from build123d import *

# Parameters (mm, degrees)
SKETCH2_R           = 1.55
BOSS_EXTRUDE1_DEPTH = 7.5
SKETCH4_W           = 8
SKETCH4_H           = 1.5
BOSS_EXTRUDE3_DEPTH = 20
SKETCH5_R           = 1.55
BOSS_EXTRUDE4_DEPTH = 7.5
SKETCH6_W           = 0.75
SKETCH6_H           = 0.5
CUT_EXTRUDE1_DEPTH  = 9
SKETCH7_R           = 1.1
CUT_EXTRUDE2_DEPTH  = 3.5
CHAMFER1_SIZE       = 1.1
FILLET1_R           = 3


with BuildPart() as part:
    # Sketch2 → Boss-Extrude1 (new body)
    with BuildSketch(Plane.XY):
        with BuildLine():
            Line((3.05, 2.05), (11.05, 2.05))
            Line((11.05, 2.05), (11.05, 0.55))
            Line((11.05, 0.55), (3.05, 0.55))
            Line((3.05, 0.55), (3.05, 0))
            ThreePointArc((3.05, 0), (0, -3.05), (-3.05, 0))
            Line((-3.05, 0), (-3.05, 2.05))
            Line((-3.05, 2.05), (-2.258317958, 2.05))
            ThreePointArc((-2.258317958, 2.05), (-1.234908904, 2.788816953), (0, 3.05))
            Line((0, 3.05), (3.05, 3.05))
            Line((3.05, 3.05), (3.05, 2.05))
        make_face()
        Circle(SKETCH2_R, mode=Mode.SUBTRACT)
    extrude(amount=BOSS_EXTRUDE1_DEPTH)

    # Sketch4 → Boss-Extrude3 (add)
    with BuildSketch(Plane.XY.offset(7.5)):
        with Locations((7.05, 1.3)):
            Rectangle(SKETCH4_W, SKETCH4_H)
    extrude(amount=BOSS_EXTRUDE3_DEPTH)

    # Sketch5 → Boss-Extrude4 (add)
    with BuildSketch(Plane.XY.offset(27.5)):
        with BuildLine():
            Line((11.05, 0.55), (11.05, 2.05))
            Line((11.05, 2.05), (3.05, 2.05))
            Line((3.05, 2.05), (3.05, 3.05))
            Line((3.05, 3.05), (0, 3.05))
            ThreePointArc((0, 3.05), (-1.234908904, 2.788816953), (-2.258317958, 2.05))
            Line((-2.258317958, 2.05), (-3.05, 2.05))
            Line((-3.05, 2.05), (-3.05, 0))
            ThreePointArc((-3.05, 0), (0, -3.05), (3.05, 0))
            Line((3.05, 0), (3.05, 0.55))
            Line((3.05, 0.55), (11.05, 0.55))
        make_face()
        Circle(SKETCH5_R, mode=Mode.SUBTRACT)
    extrude(amount=BOSS_EXTRUDE4_DEPTH)

    # Sketch6 → Cut-Extrude1 (cut, through all)
    with BuildSketch(Plane.ZY.offset(-3.05)):
        with Locations((19.4, 1.8)):
            Rectangle(SKETCH6_W, SKETCH6_H)
    extrude(amount=-CUT_EXTRUDE1_DEPTH, mode=Mode.SUBTRACT)

    # Sketch7 → Cut-Extrude2 (cut, through all)
    with BuildSketch(Plane.XZ.offset(-0.55)):
        with Locations((7.05, 25)):
            Circle(SKETCH7_R)
        with Locations((7.05, 10)):
            Circle(SKETCH7_R)
        with Locations((7.05, 31)):
            Circle(SKETCH7_R)
        with Locations((7.05, 4)):
            Circle(SKETCH7_R)
    extrude(amount=-CUT_EXTRUDE2_DEPTH, mode=Mode.SUBTRACT)

    # Chamfer1
    chamfer1_edges = [part.edges().sort_by_distance(p)[0] for p in [
        (5.95, 0.55, 10),
        (5.95, 0.55, 25),
        (5.95, 0.55, 4),
        (5.95, 0.55, 31),
    ]]
    chamfer(chamfer1_edges, length=CHAMFER1_SIZE)

    # Fillet1
    fillet1_edges = [part.edges().sort_by_distance(p)[0] for p in [
        (11.05, 1.3, 0),
        (11.05, 1.3, 35),
    ]]
    fillet(fillet1_edges, radius=FILLET1_R)


solid = part.part
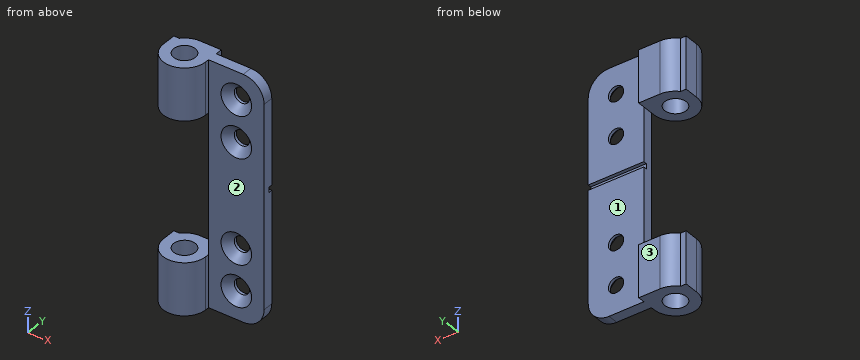
Source: CAD feature listing. Evaluate the final solid. Frame: model axes, mm. Face numbers are marked on the shaded views. A direction names the side the tool comes from. Give positions to 0.01 mm unless a question says otherwise; leave off trailing zeros. Loops run counter-clockwise (first coordinate to the right, second up) from the corner with the lowest first, then second, coordinate; pieces in that order, holes last. Notation, with made-up numbers: (-14, -38) -> (25, -38) arc R26 cw to (25, -14) -> close; hole circle Ø2 at (-25, 65.5). An arc over 180 degrees is marked (long way). Use a Markdown table: item, result. Add a question column.
1) First-contact query: pin 1 (0.8 mm diameter, centred on y = 3, z = 32, fed in from +X); pin 2 (6.5 mm diameter, centred on x = 8, z = 11.5, fed in from +Y); pin 3 (4 mm diameter, centred on x = 7.5, z = 11.5, fed in from -Y); pin 4 (1.9 mm diameter, centred on x = 0, y = 0, fed in from +Z). Flat tips, straight axial feed; report the tip coordinate or a pass-through.
2) Section query B-B, the plane x = 7.05. Count the separate pieces of the cut face and the enclosed holes in it, then the cut area to 3 significant figures.
3) Section query D-D, the plane y = 2.5. Return the cut outline in (x, z).
4) Line query: line 1 along Z through (x, y) = (7.05, 1.9) (3 decimals); line 2 along Y through (x, z) = (0, 4.5); line 3 along Z through (x, y) = (0, 2.5). Output: solid intervals per line, ascending. Write a range as [from, to].
5) Section query C-C, the plane z = 10. Return the cut outline in (x, y), then the cut area to 3 significant figures.
6) Reachability of the marked faces 1, 2 and 3 from +Z, -Z, +X, -X, +Y, -Y: full face, straight path, thin tool, end or side. Return the list, or none.
7) Section query A-A, the plane z = 31. Return the cut outline in (x, y), then the cut area to 3 significant figures.
Numbers:
| question | item | result |
|---|---|---|
| 1 | pin 1 | stops at x = 3.05 |
| 1 | pin 2 | stops at y = 2.05 |
| 1 | pin 3 | stops at y = 0.55 |
| 1 | pin 4 | passes through |
| 2 | separate pieces | 5 |
| 2 | enclosed holes | 0 |
| 2 | area | 34.1 mm2 |
| 3 | outline | (-1.75, 0) -> (3.05, 0) -> (3.05, 7.5) -> (-1.75, 7.5) -> close; (-1.75, 27.5) -> (3.05, 27.5) -> (3.05, 35) -> (-1.75, 35) -> close |
| 4 | line 1 | z = [0, 2.9], [5.1, 8.9], [11.1, 19.025], [19.775, 23.9], [26.1, 29.9], [32.1, 35] |
| 4 | line 2 | y = [-3.05, -1.55], [1.55, 3.05] |
| 4 | line 3 | z = [0, 7.5], [27.5, 35] |
| 5 | outline | (3.05, 0.55) -> (4.85, 0.55) -> (5.95, 1.65) -> (5.95, 2.05) -> (3.05, 2.05) -> close; (8.15, 1.65) -> (9.25, 0.55) -> (11.05, 0.55) -> (11.05, 2.05) -> (8.15, 2.05) -> close |
| 5 | area | 7.49 mm2 |
| 6 | face 1 | +Z, -Z, +X, +Y |
| 6 | face 2 | +Z, -Z, +X, -Y |
| 6 | face 3 | +Z, -Z, +X, -X, +Y |
| 7 | outline | (-3.05, 0) arc R3.05 ccw to (3.05, 0) -> (3.05, 0.55) -> (4.85, 0.55) -> (5.95, 1.65) -> (5.95, 2.05) -> (3.05, 2.05) -> (3.05, 3.05) -> (0, 3.05) arc R3.05 ccw to (-2.26, 2.05) -> (-3.05, 2.05) -> close; (8.15, 1.65) -> (9.25, 0.55) -> (11.05, 0.55) -> (11.05, 2.05) -> (8.15, 2.05) -> close; hole circle Ø3.1 at (0, 0) |
| 7 | area | 31.7 mm2 |
